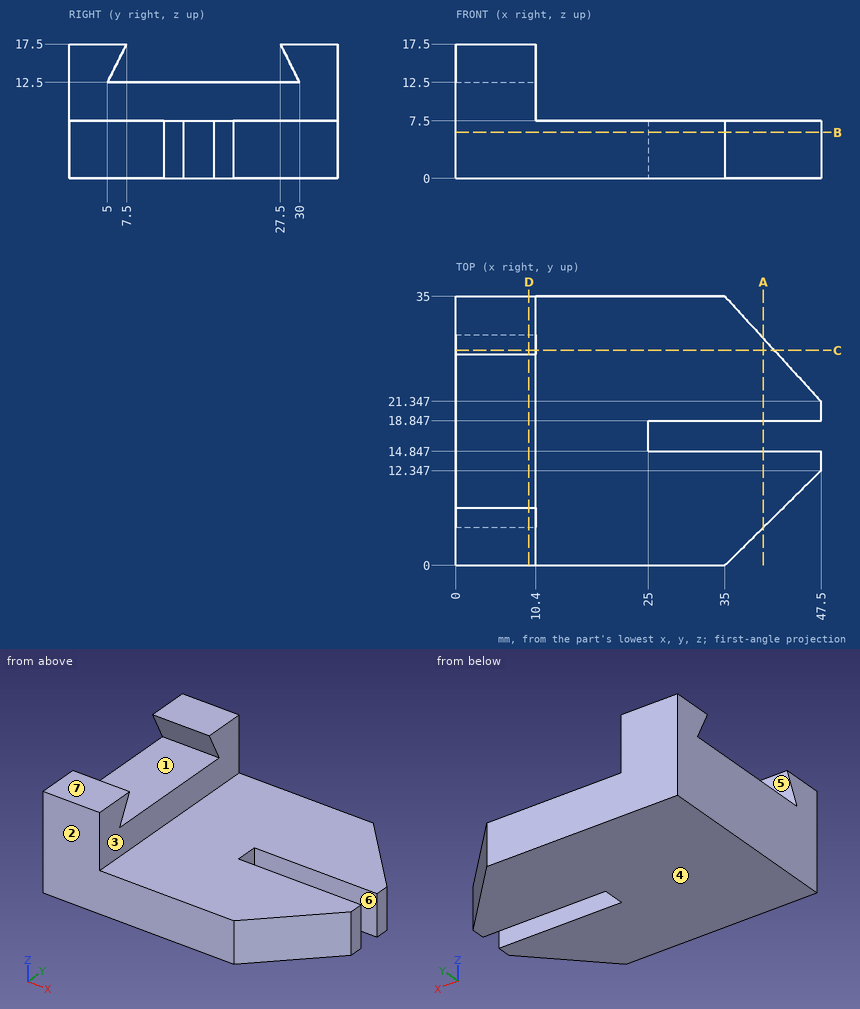
Part print with two shaded views. Sizes in mm from the minimum x, y, z corner. A direction names the side the tool comes from. Give positions to 0.01 mm unless a question says otherwise; leave off trailing zeros. Order: outer loops, then holes, each group sorted by start corner. A loop starts at its lowest first (then second) coordinate and runs counter-clockwise, first axis right, second up.
1) Saw through at B-B, the plane z = 6. Write the cut outline in (x, y).
2) 3-axis set-ups, long thin cutter, end or side, ignore diameter. For the marked faces 1, 2 and 3: which of +Z, -Z, +X, -X, +Y, -Y reach the whole face in a straight line?
3) Saw through at C-C, the plane y = 28. Write the cut outline in (x, z), then the cut area to 3 significant figures.
4) Pin check, flat tips, straight feed: pin 1 (3 mm diameter, centred on y = 6.5, z = 12.5, fed in from +X); pin 2 (12 mm diameter, centred on x = 17, y = 15, fed in from +Z); pin 3 (5 mm diameter, centred on x = 7.5, y = 15, fed in from +Z). Stop position of each tip, or through.
5) Saw through at D-D, the plane x = 9.5. Write the cut outline in (y, z), then the cut area to 3 significant figures.
6) Wall check: probe 1 along Z at (x, y) = (40.5, 27); probe 2 along Y at (x, z) = (33, 6.5); probe 3 along X at (y, z) = (8.5, 11.75). Give the ranges that are in metal, low to high.
7) Mould opens along Z. For the marked faces 4, 5, 6 and 7 say: +Z half, -Z half, draft (parallel to the pull), parting line (faces both ways), or undercut.
8) Saw through at A-A, the plane x = 40. Write the cut outline in (y, z).
Computed:
1. outline: (0, 0) - (35, 0) - (47.5, 12.35) - (47.5, 14.85) - (25, 14.85) - (25, 18.85) - (47.5, 18.85) - (47.5, 21.35) - (35, 35) - (0, 35) - close
2. face 1: +X, -X
2. face 2: +Z, -Z, +X, -X, -Y
2. face 3: +Z, +X, +Y, -Y
3. outline: (0, 0) - (41.41, 0) - (41.41, 7.5) - (10.4, 7.5) - (10.4, 12.5) - (0, 12.5) - close; (0, 16.5) - (10.4, 16.5) - (10.4, 17.5) - (0, 17.5) - close
3. area: 373 mm2
4. pin 1: stops at x = 10.4
4. pin 2: stops at z = 7.5
4. pin 3: stops at z = 12.5
5. outline: (0, 0) - (35, 0) - (35, 17.5) - (27.5, 17.5) - (30, 12.5) - (5, 12.5) - (7.5, 17.5) - (0, 17.5) - close
5. area: 500 mm2
6. probe 1: z = 0 to 7.5
6. probe 2: y = 0 to 14.85, 18.85 to 35
6. probe 3: x = 0 to 10.4
7. face 4: -Z half
7. face 5: undercut
7. face 6: draft
7. face 7: +Z half
8. outline: (4.94, 0) - (14.85, 0) - (14.85, 7.5) - (4.94, 7.5) - close; (18.85, 0) - (29.54, 0) - (29.54, 7.5) - (18.85, 7.5) - close
